Model file for the job. Use its own axes, mm. Face numbers are marked on the shaded views. A direction names the side the tool comes from. Round coordinates to 2 decimals unless told otherwise and drop trailing zeros. Loops run counter-clockwise (first coordinate to the right, second up) from the corner with the lowest first, then second, coordinate; pieces in that order, holes last. Notation, with made-up numbers: M -36.5,30 L -9.5,30 A5 cw -9.5,34 Z; hole C 18.5,76.5 d4. An arc over 180 degrees is marked long. Use a Markdown table: item, result. Add a question column.
Q1. Pin check, flat tips, straight feed: pin 1 (19 mm diameter, centred on x = 38, z = -38, fed in from +Y); pin 2 (6 mm diameter, centred on x = -38, z = -36, fed in from +Y); pin 3 (5 mm diameter, centred on y = 12, z = -4, fed in from +X). Stop position of each tip, or through.
Q2. Cut at D-D (z = 36.5). Give the cut face in (x, y), plus the area to 3 significant figures.
Q3. Cut at A-A (z = -38). Give the cut face in (x, y).
Q4. Tool access for the marked faces 3 and 4: list every direction of +Z, -Z, +X, -X, +Y, -Y with a clear straight run to the whole face (end or side of a thin tool).
Q5. Cut at C-C (y = 10). Give the cut face in (x, z).
Q6. Mould opens along Z. For the marked faces 1 and 2 say: +Z half, -Z half, draft (parallel to the pull), parting line (faces both ways), or undercut.
Q7. Probe line 1 (X direction, y = 4.8, z = -38); line 2 (Z direction, x = -18, y = 6.75); line 3 (X direction, y = 12.1, z = 0). List the from-to ranges inside material, lowest first. Write a range as from..to.
Q8. Cut at B-B (x = 0). Give the cut face in (y, z), plus the area to 3 significant figures.
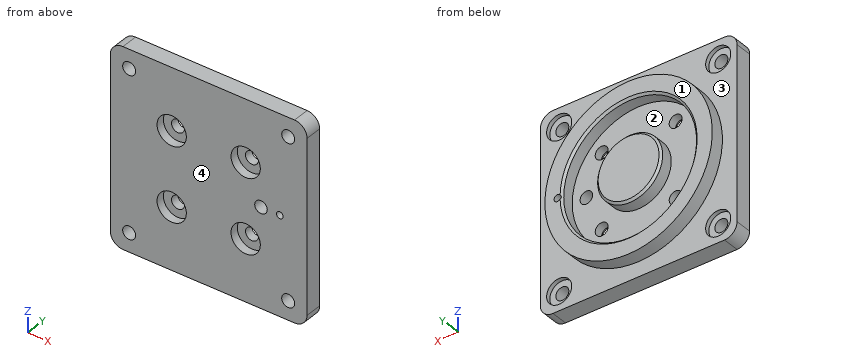
from build123d import *

# Parameters (mm, degrees)
SKETCH1_W           = 94
SKETCH1_H           = 94
SKETCH1_R           = 1.6
SKETCH1_R_2         = 3.1
SKETCH1_R_3         = 3
BOSS_EXTRUDE1_DEPTH = 8
SKETCH2_R           = 7
CUT_EXTRUDE1_DEPTH  = 4
SKETCH3_R           = 40
SKETCH3_R_2         = 1.6
SKETCH3_R_3         = 31.75
SKETCH3_R_4         = 15.55
BOSS_EXTRUDE2_DEPTH = 6.4
CHAMFER1_SIZE       = 1
FILLET1_R           = 6
SKETCH5_R           = 3.1
CUT_EXTRUDE2_DEPTH  = 67.947740825
SKETCH6_R           = 6
CUT_EXTRUDE3_DEPTH  = 2


with BuildPart() as part:
    # Sketch1 → Boss-Extrude1 (new body)
    with BuildSketch(Plane(origin=(0, 0, 0), x_dir=(1, 0, 0), z_dir=(0, 1, 0))):
        Rectangle(SKETCH1_W, SKETCH1_H)
        with Locations(Location((34, 0, 0), (0, 0, 270))):
            Circle(SKETCH1_R, mode=Mode.SUBTRACT)
        with Locations(Location((17.67766953, -17.67766953, 0), (0, 0, 270))):
            Circle(SKETCH1_R_2, mode=Mode.SUBTRACT)
        with Locations(Location((25, 0, 0), (0, 0, 270))):
            Circle(SKETCH1_R_3, mode=Mode.SUBTRACT)
        with Locations(Location((-17.67766953, -17.67766953, 0), (0, 0, 270))):
            Circle(SKETCH1_R_2, mode=Mode.SUBTRACT)
        with Locations(Location((-17.67766953, 17.67766953, 0), (0, 0, 270))):
            Circle(SKETCH1_R_2, mode=Mode.SUBTRACT)
        with Locations(Location((17.67766953, 17.67766953, 0), (0, 0, 270))):
            Circle(SKETCH1_R_2, mode=Mode.SUBTRACT)
    extrude(amount=BOSS_EXTRUDE1_DEPTH)

    # Sketch2 → Cut-Extrude1 (cut)
    with BuildSketch(Plane.XZ):
        with Locations(Location((17.67766953, 17.67766953, 0), (0, 0, 270))):
            Circle(SKETCH2_R)
        with Locations(Location((17.67766953, -17.67766953, 0), (0, 0, 270))):
            Circle(SKETCH2_R)
        with Locations(Location((-17.67766953, -17.67766953, 0), (0, 0, 270))):
            Circle(SKETCH2_R)
        with Locations(Location((-17.67766953, 17.67766953, 0), (0, 0, 270))):
            Circle(SKETCH2_R)
    extrude(amount=-CUT_EXTRUDE1_DEPTH, mode=Mode.SUBTRACT)

    # Sketch3 → Boss-Extrude2 (add)
    # profile 1 of 2: a face of its own
    with BuildSketch(Plane(origin=(0, 8, 0), x_dir=(1, 0, 0), z_dir=(0, 1, 0))):
        with Locations(Location((0, 0, 0), (0, 0, 270))):
            Circle(SKETCH3_R)
        with Locations(Location((34, 0, 0), (0, 0, 270))):
            Circle(SKETCH3_R_2, mode=Mode.SUBTRACT)
        with Locations(Location((0, 0, 0), (0, 0, 270))):
            Circle(SKETCH3_R_3, mode=Mode.SUBTRACT)
    # profile 2 of 2: a face of its own
    with BuildSketch(Plane(origin=(0, 8, 0), x_dir=(1, 0, 0), z_dir=(0, 1, 0))):
        with Locations(Location((0, 0, 0), (0, 0, 270))):
            Circle(SKETCH3_R_4)
    extrude(amount=BOSS_EXTRUDE2_DEPTH)

    # Chamfer1
    # the kernel refuses this chamfer: 1 mm, written as the material it takes off along each edge
    with BuildSketch(Plane(origin=(0, 14.4, 0), x_dir=(0, 0, 1), z_dir=(-1, 0, 0))) as chamfer1_piece_1:
        Polygon((15.55, -CHAMFER1_SIZE), (15.55 - CHAMFER1_SIZE, 0), (15.55, 0), align=None)
    revolve(axis=Axis((0, 14.4, 0), (0, 1, 0)), mode=Mode.SUBTRACT)
    with BuildSketch(Plane(origin=(0, 14.4, 0), x_dir=(0, 0, 1), z_dir=(-1, 0, 0))) as chamfer1_piece_2:
        Polygon((31.75 + CHAMFER1_SIZE, 0), (31.75, -CHAMFER1_SIZE), (31.75, 0), align=None)
    revolve(axis=Axis((0, 14.4, 0), (0, 1, 0)), mode=Mode.SUBTRACT)

    # Fillet1
    fillet1_edges = [part.edges().sort_by_distance(p)[0] for p in [
        (47, 4, 47),
        (-47, 4, 47),
        (-47, 4, -47),
        (47, 4, -47),
    ]]
    fillet(fillet1_edges, radius=FILLET1_R)

    # Sketch5 → Cut-Extrude2 (cut, through all)
    with BuildSketch(Plane(origin=(0, 8, 0), x_dir=(1, 0, 0), z_dir=(0, 1, 0))):
        with Locations(Location((-38, 38, 0), (0, 0, 270))):
            Circle(SKETCH5_R)
        with Locations(Location((38, 38, 0), (0, 0, 270))):
            Circle(SKETCH5_R)
        with Locations(Location((38, -38, 0), (0, 0, 270))):
            Circle(SKETCH5_R)
        with Locations(Location((-38, -38, 0), (0, 0, 270))):
            Circle(SKETCH5_R)
    extrude(amount=-CUT_EXTRUDE2_DEPTH, mode=Mode.SUBTRACT)

    # Sketch6 → Cut-Extrude3 (cut)
    with BuildSketch(Plane(origin=(0, 8, 0), x_dir=(1, 0, 0), z_dir=(0, 1, 0))):
        with Locations(Location((-38, 38, 0), (0, 0, 270))):
            Circle(SKETCH6_R)
        with Locations(Location((38, 38, 0), (0, 0, 270))):
            Circle(SKETCH6_R)
        with Locations(Location((38, -38, 0), (0, 0, 270))):
            Circle(SKETCH6_R)
        with Locations(Location((-38, -38, 0), (0, 0, 270))):
            Circle(SKETCH6_R)
    extrude(amount=-CUT_EXTRUDE3_DEPTH, mode=Mode.SUBTRACT)


solid = part.part
Checked values:
| question | item | result |
|---|---|---|
| 1 | pin 1 | stops at y = 8 |
| 1 | pin 2 | stops at y = 6 |
| 1 | pin 3 | stops at x = 39.97 |
| 2 | outline | M -47,0 L -40.71,0 L -40.71,6 L -43.81,6 L -43.81,8 L -47,8 Z; M -35.29,0 L 35.29,0 L 35.29,6 L 32.19,6 L 32.19,8 L 16.36,8 L 16.36,14.4 L -16.36,14.4 L -16.36,8 L -32.19,8 L -32.19,6 L -35.29,6 Z; M 40.71,0 L 47,0 L 47,8 L 43.81,8 L 43.81,6 L 40.71,6 Z |
| 2 | area | 850 mm^2 |
| 3 | outline | M -47,0 L -41.1,0 L -41.1,6 L -44,6 L -44,8 L -47,8 Z; M -34.9,0 L 34.9,0 L 34.9,6 L 32,6 L 32,8 L 12.49,8 L 12.49,14.4 L -12.49,14.4 L -12.49,8 L -32,8 L -32,6 L -34.9,6 Z; M 41.1,0 L 47,0 L 47,8 L 44,8 L 44,6 L 41.1,6 Z |
| 4 | face 3 | +Y |
| 4 | face 4 | +Z, -Z, +X, -X, -Y |
| 5 | outline | C 0,0 d80; C 0,0 d31.1; hole C 0,0 d63.5; hole C 34,0 d3.2 |
| 6 | face 1 | draft |
| 6 | face 2 | undercut |
| 7 | line 1 | x = -47..-41.1, -34.9..34.9, 41.1..47 |
| 7 | line 2 | z = -47..-20.76, -14.59..14.59, 20.76..47 |
| 7 | line 3 | x = -40..-31.75, -15.55..15.55, 31.75..32.4, 35.6..40 |
| 8 | outline | M 0,-47 L 8,-47 L 8,-40 L 14.4,-40 L 14.4,-32.75 L 13.4,-31.75 L 8,-31.75 L 8,-15.55 L 13.4,-15.55 L 14.4,-14.55 L 14.4,14.55 L 13.4,15.55 L 8,15.55 L 8,31.75 L 13.4,31.75 L 14.4,32.75 L 14.4,40 L 8,40 L 8,47 L 0,47 Z |
| 8 | area | 1,050 mm^2 |
